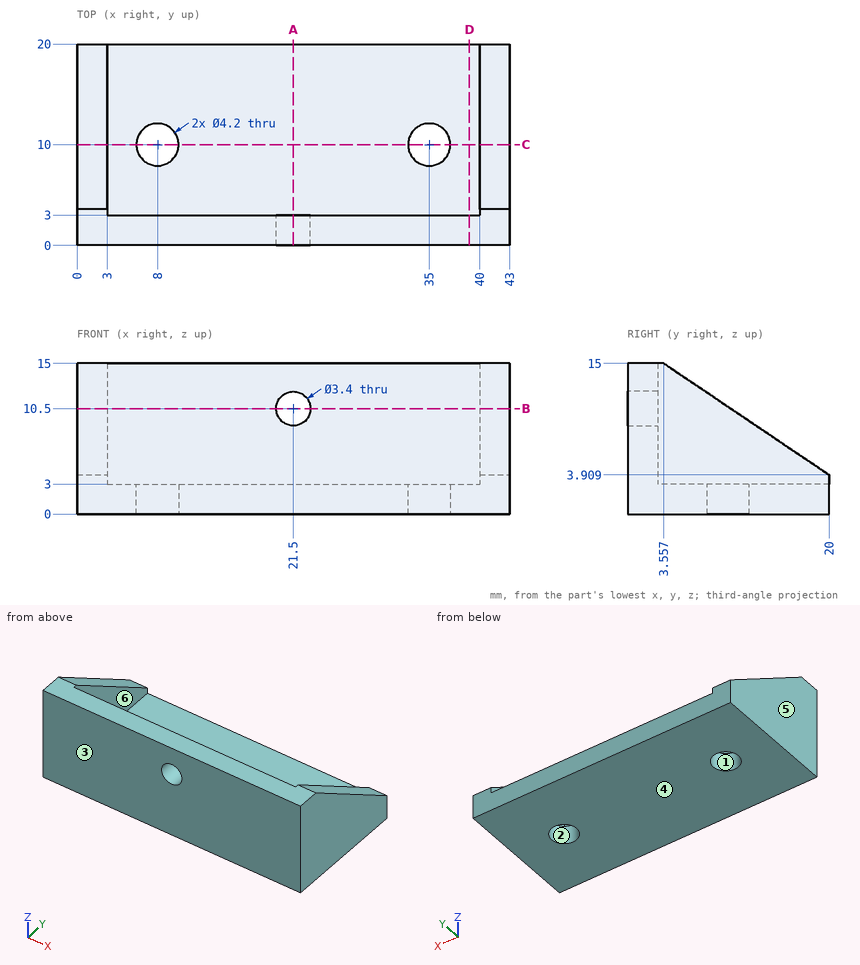
Answer from the drawing. Dimensions are ordinates in mm from the lowest x, y and z of the part. A direction names the side the tool comes from. Coordinates: 2 decimals unless noted, no trailing zeros. Order: outer loops, then holes, each group sorted by start corner. A loop starts at its lowest first (then second) coordinate and runs counter-clockwise, first axis right, second up. Notation, with made-up numbers: (39.25, -27.5) - (97.25, -27.5) arc R21 ccw to (97.25, 8.5) - close; hole circle Ø6 at (26.5, 26). An arc over 180 degrees is marked (long way). Put each result on its own line as item: value. Start each with the question number.
1) Find the intervals of material crossed by line 1 (X direction, y = 11.5, z = 6); line 2 (X direction, y = 2.3, z = 10.5); line 3 (Z direction, x = 35, y = 5.5), in increasing order. Write a range as from..to.
2) For a pull along Y with two mould halves and no side action, classify the marked faces 1, 2, 3 and 4 as released by +Y, released by -Y, zero draft, split by the parting line, or undercut.
3) Find section A-A (x = 21.5). Give the vertices of the cut face in (y, z).
4) For the marked faces 5 and 6, determine the directions among +Z, -Z, +X, -X, +Y, -Y from which every point of the face is accessible in a straight line to the end or side of a thin tool.
5) Find section C-C (y = 10). Give the vertices of the cut face in (x, z), plus the area to 3 significant figures.
6) Flat-ended cylindrical pins translate along their axes: pin 1 (1.5 mm diameter, centred on x = 29.5, z = 2, fed in from -Y); pin 2 (2 mm diameter, centred on x = 26, y = 7.5, fed in from +Z); pin 3 (3 mm diameter, centred on x = 21.5, z = 10.5, fed in from -Y). Find the tip coordinate at first contact, or state that the pin passes through.
7) Find section B-B (z = 10.5). Give the vertices of the cut face in (x, y), plus the area to 3 significant figures.
8) Find section D-D (x = 39). Give the vertices of the cut face in (y, z), plus the area to 3 significant figures.
Results list:
1. line 1: x = 0..3, 40..43
1. line 2: x = 0..19.8, 23.2..43
1. line 3: z = 0..3
2. face 1: undercut
2. face 2: undercut
2. face 3: released by -Y
2. face 4: zero draft
3. outline: (0, 0) - (20, 0) - (20, 3) - (3, 3) - (3, 8.8) - (0, 8.8) - close; (0, 12.2) - (3, 12.2) - (3, 15) - (0, 15) - close
4. face 5: +Z, -Z, -X, +Y, -Y
4. face 6: +Z, +Y
5. outline: (0, 0) - (5.9, 0) - (5.9, 3) - (3, 3) - (3, 10.65) - (0, 10.65) - close; (10.1, 0) - (32.9, 0) - (32.9, 3) - (10.1, 3) - close; (37.1, 0) - (43, 0) - (43, 10.65) - (40, 10.65) - (40, 3) - (37.1, 3) - close
5. area: 150 mm^2
6. pin 1: stops at y = 0
6. pin 2: stops at z = 3
6. pin 3: passes through
7. outline: (0, 0) - (19.8, 0) - (19.8, 3) - (3, 3) - (3, 10.23) - (0, 10.23) - close; (23.2, 0) - (43, 0) - (43, 10.23) - (40, 10.23) - (40, 3) - (23.2, 3) - close
7. area: 162 mm^2
8. outline: (0, 0) - (20, 0) - (20, 3) - (3, 3) - (3, 15) - (0, 15) - close
8. area: 96.0 mm^2
